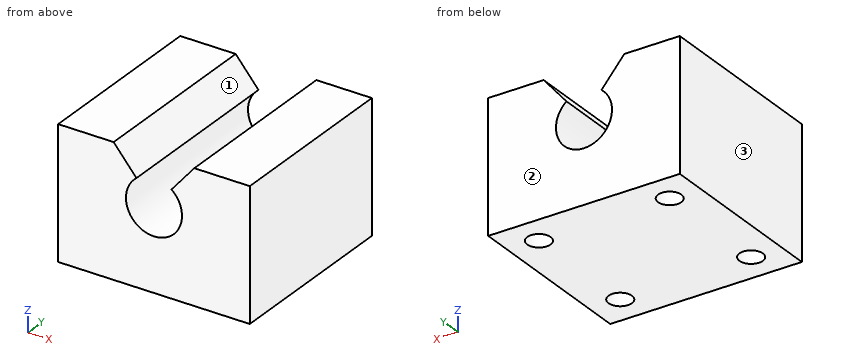
from build123d import *

# Parameters (mm, degrees)
SKETCH1_W               = 41
SKETCH1_H               = 28
SKETCH1_R               = 6
BOSS_EXTRUDE1_DEPTH     = 39
CUT_EXTRUDE1_DEPTH      = 1
CUT_EXTRUDE1_DEPTH_BACK = 40
SKETCH3_R               = 2.5
CUT_EXTRUDE2_DEPTH      = 10


with BuildPart() as part:
    # Sketch1 → Boss-Extrude1 (new body)
    with BuildSketch(Plane(origin=(0, 0, 0), x_dir=(1, 0, 0), z_dir=(0, 1, 0))):
        with Locations((0, 3.5)):
            Rectangle(SKETCH1_W, SKETCH1_H)
        Circle(SKETCH1_R, mode=Mode.SUBTRACT)
    extrude(amount=BOSS_EXTRUDE1_DEPTH)

    # Sketch2 → Cut-Extrude1 (cut, two sides)
    with BuildSketch(Plane(origin=(0, 39, 0), x_dir=(1, 0, 0), z_dir=(0, 1, 0))) as cut_extrude1_sk:
        with BuildLine():
            ThreePointArc((3.75, -4.683748499), (0, -6), (-3.75, -4.683748499))
            Line((-3.75, -4.683748499), (-8.630414489, -10.5))
            Line((-8.630414489, -10.5), (8.630414489, -10.5))
            Line((8.630414489, -10.5), (3.75, -4.683748499))
        make_face()
    extrude(amount=CUT_EXTRUDE1_DEPTH, mode=Mode.SUBTRACT)
    extrude(cut_extrude1_sk.sketch, amount=-CUT_EXTRUDE1_DEPTH_BACK, mode=Mode.SUBTRACT)

    # Sketch3 → Cut-Extrude2 (cut)
    with BuildSketch(Plane(origin=(0, 0, -17.5), x_dir=(-1, 0, 0), z_dir=(0, 0, -1))):
        with Locations((14, 32.5)):
            Circle(SKETCH3_R)
        with Locations((-14, 6.5)):
            Circle(SKETCH3_R)
        with Locations((-14, 32.5)):
            Circle(SKETCH3_R)
        with Locations((14, 6.5)):
            Circle(SKETCH3_R)
    extrude(amount=-CUT_EXTRUDE2_DEPTH, mode=Mode.SUBTRACT)


solid = part.part
Read the model definition and answer for the solid it produces. Units are mm, in the model's axes. Face numbers are marked on the shaded views. Round coordinates to 2 decimals unless told otherwise and drop trailing zeros. Write each loop counter-clockwise with the first axis right and the second up, starting at its lowest first coordinate (ties: lowest second). Pieces come first, ordered by that corner, then holes.
1. The part is cut by section D-D, the plane x = 14. Determine the outline of the cut face in (y, z), then the cut area to 3 significant figures.
2. The part is cut by section A-A, the plane z = 0. Determine the outline of the cut face in (x, y).
3. The part is cut by section B-B, the plane y = 36. Determine the outline of the cut face in (x, z), then the cut area to 3 significant figures.
4. The part is cut by section C-C, the plane z = -10.5. Determine the outline of the cut face in (x, y).
5. Straight lines are drawn through the part: L1, parallel to Y at x = 14, z = -12.5; L2, parallel to X at y = 26, z = -0.25; L3, parallel to X at y = 11, z = -1. For each, find the intervals that lie inside material, in ascending order.
6. Determine the mould class of the marked faces 1, 2 and 3 for opening direction X: pulls with the +X half, pulls with the -X half, needs draft (parallel to the pull), parting line crosses it, or undercut.
7. Given pin 1 Ø3 at (x, y) = (14, 32.5) entering from -Z; pin 2 Ø1 at (x, z) = (10, -11.5) entering from -Y, each flat-ended and moving along its own axis, determine where each tip first touches the part or whether it passes through.
Values:
1. outline: (0, -17.5) - (4, -17.5) - (4, -7.5) - (9, -7.5) - (9, -17.5) - (30, -17.5) - (30, -7.5) - (35, -7.5) - (35, -17.5) - (39, -17.5) - (39, 10.5) - (0, 10.5) - close
1. area: 992 mm2
2. outline: (-20.5, 0) - (-6, 0) - (-6, 39) - (-20.5, 39) - close; (6, 0) - (20.5, 0) - (20.5, 39) - (6, 39) - close
3. outline: (-20.5, -17.5) - (20.5, -17.5) - (20.5, 10.5) - (8.63, 10.5) - (3.75, 4.68) arc R6 cw (long way) to (-3.75, 4.68) - (-8.63, 10.5) - (-20.5, 10.5) - close
3. area: 970 mm2
4. outline: (-20.5, 0) - (20.5, 0) - (20.5, 39) - (-20.5, 39) - close; hole circle Ø5 at (-14, 6.5); hole circle Ø5 at (-14, 32.5); hole circle Ø5 at (14, 6.5); hole circle Ø5 at (14, 32.5)
5. L1: y = 0 to 4, 9 to 30, 35 to 39
5. L2: x = -20.5 to -5.99, 5.99 to 20.5
5. L3: x = -20.5 to -5.92, 5.92 to 20.5
6. face 1: undercut
6. face 2: needs draft
6. face 3: pulls with the -X half
7. pin 1: stops at z = -7.5
7. pin 2: stops at y = 0
